from build123d import *

# Parameters (mm, degrees)
F0_R     = 8.4455
F1_DEPTH = 6.35
F2_R     = 11.718365
F3_DEPTH = 6.35
F4_R     = 3.175
F5_DEPTH = 57.15


with BuildPart() as f1:
    # F0 (on Front) → F1 (new body)
    with BuildSketch(Plane.XZ):
        Circle(F0_R)
    extrude(amount=F1_DEPTH)

    # F2 (on Front) → F3 (join)
    with BuildSketch(Plane.XZ):
        Circle(F2_R)
    extrude(amount=-F3_DEPTH)

    # F4 (on Front) → F5 (join)
    with BuildSketch(Plane.XZ):
        Circle(F4_R)
    extrude(amount=-F5_DEPTH)


solid = f1.part
Input: part model. Units: mm. Frame: model coordinates. A direction names the side the tool comes from. Give positions to 0.01 mm unless a question says otherwise; leave off trailing zeros. Order: outer loops, then holes, each group sorted by start corner. A loop starts at its lowest first (then second) coordinate and runs counter-clockwise, first axis right, second up. Notation, with made-up numbers: M 0.25,-23 L 44.25,-23 A35 cw 44.25,16 Z; hole C 65,8.5 d9. An arc over 180 degrees is marked long. Answer as a JSON object with one key per item and string values.
1. First-contact query: P1, Ø2, axis at y = 18, z = -5.5, coming from the +X side; P2, Ø10, axis at x = 3, y = 39, coming from the -Z side (3 decimals); P3, Ø4, axis at x = -3, z = -9, coming from the +Y side. Flat tips, straight axial feed; report the tip coordinate or a pass-through.
Result sheet:
{"P1": "through", "P2": "z = -3.175", "P3": "y = 6.35"}
2. Cut plane C-C, the plane y = 7.5. Output: boundary loops of the cut face in (x, z) (3 decimals), and give its area (3 significant figures).
Result sheet:
{"outline": "C 0,0 d6.35", "area": "31.7 mm²"}
3. Cut plane D-D, the plane x = -6.25. Output: boundary loops of the cut face in (y, z), and give its area (3 significant figures).
Result sheet:
{"outline": "M -6.35,-5.68 L 0,-5.68 L 0,-9.91 L 6.35,-9.91 L 6.35,9.91 L 0,9.91 L 0,5.68 L -6.35,5.68 Z", "area": "198 mm²"}
4. Reachability of faces 1 (the flat face through (2.4, 6.35, -2.4)), 2 (the flat face through (0, -6.35, 0)), 3 (the cylindrical face through (8.056, -3.131, 2.537)) from +Z, -Z, +X, -X, +Y, -Y: full face, straight path, thin tool, end or side. Return the list, or none.
Result sheet:
{"face 1": "+Y", "face 2": "+Z, -Z, +X, -X, -Y", "face 3": "-Y"}
5. Ray query, line 1 (Y direction, x = 1.25, z = -7.75); line 2 (Z direction, x = 0.25, y = 49.5); line 3 (Y direction, x = -8.75, z = 6.75). Return the intervals inside material, ascending. Write a range as [from, to].
Result sheet:
{"line 1": "[-6.35, 6.35]", "line 2": "[-3.17, 3.17]", "line 3": "[0, 6.35]"}
